```python
from build123d import *

# Parameters (mm, degrees)
CROQUIS1_R                   = 9
CROQUIS1_R_2                 = 1.5
SALIENTE_EXTRUIR1_DEPTH      = 15
SALIENTE_EXTRUIR1_DEPTH_BACK = 8
CROQUIS2_R                   = 9
CROQUIS2_R_2                 = 2.4
SALIENTE_EXTRUIR4_DEPTH      = 20
CROQUIS7_R                   = 2.4
CORTAR_EXTRUIR1_DEPTH        = 20
CROQUIS8_R                   = 1.5
CORTAR_EXTRUIR2_DEPTH        = 15
CROQUIS9_R                   = 1.4
CORTAR_EXTRUIR3_DEPTH        = 19
CROQUIS10_R                  = 1.4
CORTAR_EXTRUIR4_DEPTH        = 1
CORTAR_EXTRUIR4_DEPTH_BACK   = 33.0000001


with BuildPart() as part:
    # Croquis1 → Saliente-Extruir1 (new body, two sides)
    with BuildSketch(Plane.XY) as saliente_extruir1_sk:
        Circle(CROQUIS1_R)
        Circle(CROQUIS1_R_2, mode=Mode.SUBTRACT)
    extrude(amount=SALIENTE_EXTRUIR1_DEPTH)
    extrude(saliente_extruir1_sk.sketch, amount=-SALIENTE_EXTRUIR1_DEPTH_BACK)

    # Croquis2 → Saliente-Extruir4 (add)
    with BuildSketch(Plane(origin=(0, 0, 0), x_dir=(1, 0, 0), z_dir=(0, 1, 0))):
        with Locations((0, 8)):
            Circle(CROQUIS2_R)
        with Locations((0, 8)):
            Circle(CROQUIS2_R_2, mode=Mode.SUBTRACT)
    extrude(amount=SALIENTE_EXTRUIR4_DEPTH)

    # Croquis6 → Revolución4 (revolve)
    with BuildSketch(Plane(origin=(0, 0, -8), x_dir=(-1, 0, 0), z_dir=(0, 0, -1))):
        with BuildLine():
            Line((0, 0), (0, -9))
            ThreePointArc((0, -9), (-6.363961031, -6.363961031), (-9, 0))
            Line((-9, 0), (0, 0))
        make_face()
    revolve(axis=Axis((0, 0, -8), (0, -1, 0)))

    # Croquis7 → Cortar-Extruir1 (cut)
    with BuildSketch(Plane(origin=(0, 20, 0), x_dir=(1, 0, 0), z_dir=(0, 1, 0))):
        with Locations((0, 8)):
            Circle(CROQUIS7_R)
    extrude(amount=-CORTAR_EXTRUIR1_DEPTH, mode=Mode.SUBTRACT)

    # Croquis8 → Cortar-Extruir2 (cut)
    with BuildSketch(Plane.XY.offset(15)):
        Circle(CROQUIS8_R)
    extrude(amount=-CORTAR_EXTRUIR2_DEPTH, mode=Mode.SUBTRACT)

    # Croquis9 → Cortar-Extruir3 (cut, through all)
    with BuildSketch(Plane.ZY.offset(9)):
        with Locations((8, 0)):
            Circle(CROQUIS9_R)
    extrude(amount=-CORTAR_EXTRUIR3_DEPTH, mode=Mode.SUBTRACT)

    # Croquis10 → Cortar-Extruir4 (cut, two sides)
    with BuildSketch(Plane(origin=(0, 0, -17), x_dir=(-1, 0, 0), z_dir=(0, 0, -1))) as cortar_extruir4_sk:
        with Locations((0, 13.459047629)):
            Circle(CROQUIS10_R)
    extrude(amount=CORTAR_EXTRUIR4_DEPTH, mode=Mode.SUBTRACT)
    extrude(cortar_extruir4_sk.sketch, amount=-CORTAR_EXTRUIR4_DEPTH_BACK, mode=Mode.SUBTRACT)


solid = part.part
```
Check sheet for the modelled part. Datum: model origin and axes. Units: mm. A direction names the side the tool comes from. Coordinates: 2 decimals unless noted, no trailing zeros. Loops run counter-clockwise (first coordinate to the right, second up) from the corner with the lowest first, then second, coordinate; pieces in that order, holes last. Notation, with made-up numbers: M 68,5 L 88,5 A7 ccw 88,16 Z; hole C 63,53 d11. An arc over 180 degrees is marked long. Answer as a JSON object with one key per item and string values.
1. Sectioned sample at B-B on y = 13. Record the cut outline in (x, z), and give its area (3 significant figures).
Outcome:
{"outline": "M -1.32,-16.9 L -1.32,-10 A2.4 cw -1.32,-6 L -1.32,0.9 A9 ccw Z; M 1.32,-16.9 A9 ccw 1.32,0.9 L 1.32,-6 A2.4 cw 1.32,-10 Z", "area": "201 mm²"}
2. Sectioned sample at C-C on z = 8. Record the cut outline in (x, y).
Outcome:
{"outline": "M -8.89,-1.4 A9 ccw 8.89,-1.4 L 0.54,-1.4 A1.5 cw -0.54,-1.4 Z; M -8.89,1.4 L -0.54,1.4 A1.5 cw 0.54,1.4 L 8.89,1.4 A9 ccw Z"}
3. Depth check by flat-ended pin: P1, Ø1, axis at x = 1.5, z = -12, coming from the -Y side; P2, Ø4, axis at y = -5.5, z = -13, coming from the +X side; P3, Ø4, axis at y = 6.5, z = -1.5, coming from the -X side. Enter the tip coordinate at first touch or a pass-through.
Outcome:
{"P1": "y = -8.17", "P2": "x = 7.18", "P3": "x = -7.79"}
4. Release check for a two-part mould opening along Y. For faces 1 (the cylindrical face through (-1.951, -8.786, 3.661)), 2 (the flat face through (0, -2, 15)), 3 (the cylindrical face through (-4.83, -0.54, 9.29)) record: pulls with the +Y half, pulls with the -Y half, needs draft (parallel to the pull), parting line crosses it, or undercut.
Outcome:
{"face 1": "parting line crosses it", "face 2": "needs draft", "face 3": "undercut"}
5. Sectioned sample at D-D on x = -5.5. Record the cut outline in (y, z), and give its area (3 significant figures).
Outcome:
{"outline": "M -7.12,-8 A7.12 ccw 0,-15.12 L 20,-15.12 L 20,-0.88 L 7.12,-0.88 L 7.12,15 L -7.12,15 Z; hole C 0,8 d2.8", "area": "596 mm²"}
6. Sectioned sample at A-A on x = 0. Record the cut outline in (y, z).
Outcome:
{"outline": "M -9,-8 A9 ccw 0,-17 L 12.06,-17 L 12.06,-10.4 L 0,-10.4 L 0,-5.6 L 12.06,-5.6 L 12.06,1 L 9,1 L 9,15 L 1.5,15 L 1.5,0 L -1.5,0 L -1.5,15 L -9,15 Z; M 14.86,-17 L 20,-17 L 20,-10.4 L 14.86,-10.4 Z; M 14.86,-5.6 L 20,-5.6 L 20,1 L 14.86,1 Z"}
7. Scan lines: L1, parallel to Y at x = 0, z = -3; L2, parallel to Z at x = 0, y = 10.25; L3, parallel to Y at x = 0, z = 7.75. Record each from-to range of solid material in increasing order. Write a range as from..to.
Outcome:
{"L1": "-9..12.06, 14.86..20", "L2": "-17..-10.4, -5.6..1", "L3": "-9..-1.5, 1.5..9"}
8. Access from +Z, -Z, +X, -X, +Y, -Y to the whole of each face (thin tool, end or side, straight path). Record for faces 4 (the cylindrical face through (-0.65, 12.22, -13.52)), 5 (the cylindrical face through (-0.31, 9.86, -10.38)), 6 (the flat face through (0, 0, 0)).
Outcome:
{"face 4": "+Z, -Z", "face 5": "+Y", "face 6": "+Z"}
